from build123d import *

# Parameters (mm, degrees)
SKETCH1_R           = 2.5
BOSS_EXTRUDE1_DEPTH = 3
SKETCH2_W           = 5
SKETCH2_H           = 1
BOSS_EXTRUDE2_DEPTH = 3
CUT_EXTRUDE1_REACH  = 15.032
SKETCH3_W           = 1
SKETCH3_H           = 3.5


with BuildPart() as part:
    # Sketch1 → Boss-Extrude1 (new body)
    with BuildSketch(Plane.XY):
        with BuildLine():
            Line((-6.654411765, -2.5), (-11.654411765, -2.5))
            Line((-11.654411765, -2.5), (-11.654411765, -5))
            Line((-11.654411765, -5), (-5.608785246, -5))
            add(Edge.make_bspline(
                [(-5.608785246, -5), (3.217675956, -4.682890968), (11.654411765, -2.5)],
                knots=[0.187203543, 0.187203543, 0.187203543, 0.737930507, 0.737930507, 0.737930507], degree=2))
            Line((11.654411765, -2.5), (11.654411765, 2.5))
            add(Edge.make_bspline(
                [(-5.608785246, 5), (3.217675956, 4.682890968), (11.654411765, 2.5)],
                knots=[0.187203543, 0.187203543, 0.187203543, 0.737930507, 0.737930507, 0.737930507], degree=2))
            Line((-5.608785246, 5), (-11.654411765, 5))
            Line((-11.654411765, 5), (-11.654411765, 2.5))
            Line((-11.654411765, 2.5), (-6.654411765, 2.5))
            Line((-6.654411765, 2.5), (-6.654411765, -2.5))
        make_face()
        with Locations((6.654411765, 0)):
            Circle(SKETCH1_R, mode=Mode.SUBTRACT)
    extrude(amount=BOSS_EXTRUDE1_DEPTH)

    # Sketch2 → Boss-Extrude2 (add)
    with BuildSketch(Plane.XY.offset(3)):
        with Locations((-9.154411765, 2)):
            Rectangle(SKETCH2_W, SKETCH2_H)
        with Locations((-9.154411765, -2)):
            Rectangle(SKETCH2_W, SKETCH2_H)
    extrude(amount=-BOSS_EXTRUDE2_DEPTH)

    # Sketch3 → Cut-Extrude1 (cut, up to next)
    with BuildSketch(Plane.XY.offset(3), mode=Mode.PRIVATE) as cut_extrude1_sk1:
        with Locations((-11.154411765, 3.25)):
            Rectangle(SKETCH3_W, SKETCH3_H)
    cut_extrude1_tool1 = extrude(cut_extrude1_sk1.sketch, amount=-CUT_EXTRUDE1_REACH, mode=Mode.PRIVATE) & part.part
    # Sketch3 → Cut-Extrude1 (cut, up to next)
    with BuildSketch(Plane.XY.offset(3), mode=Mode.PRIVATE) as cut_extrude1_sk2:
        with Locations((-11.154411765, -3.25)):
            Rectangle(SKETCH3_W, SKETCH3_H)
    cut_extrude1_tool2 = extrude(cut_extrude1_sk2.sketch, amount=-CUT_EXTRUDE1_REACH, mode=Mode.PRIVATE) & part.part
    add(cut_extrude1_tool1.solids().sort_by_distance((-11.154412, 3.25, 3))[0], mode=Mode.SUBTRACT)
    add(cut_extrude1_tool2.solids().sort_by_distance((-11.154412, -3.25, 3))[0], mode=Mode.SUBTRACT)


solid = part.part
Input: part model. Units: mm. Frame: model coordinates. A direction names the side the tool comes from. Round coordinates to 2 decimals unless told otherwise and drop trailing zeros. Order: outer loops, then holes, each group sorted by start corner. A loop starts at its lowest first (then second) coordinate and runs counter-clockwise, first axis right, second up. Notation, with made-up numbers: (78.25, 40.5) - (118.25, 40.5) arc R14 ccw to (118.25, 64.5) - close; hole circle Ø7 at (24, 14). An arc over 180 degrees is marked (long way). Use a Markdown table: item, result.
1. Material intervals for probe 1 along Y at (x, z) = (-7, 2.45); probe 2 along Y at (x, z) = (-5.5, 2.25); probe 3 along X at (y, z) = (2.25, 0.75), sorted ascending.
Evaluation:
| item | result |
|---|---|
| probe 1 | -5 to -1.5, 1.5 to 5 |
| probe 2 | -5 to 5 |
| probe 3 | -10.65 to 5.56, 7.74 to 11.65 |
2. Section B-B on y = 1.25. Return the cut outline in (x, z).
Evaluation:
| item | result |
|---|---|
| outline | (-6.65, 0) - (4.49, 0) - (4.49, 3) - (-6.65, 3) - close; (8.82, 0) - (11.65, 0) - (11.65, 3) - (8.82, 3) - close |
3. Mould query, pull axis Y, two halves, no side actions, for faces 1 (the face through (11.654, 0, 1)), 2 (the face through (-8, -5, 1)), 3 (the face through (-6.654, 0, 1)). Classes: +Y half, -Y half, draft (parallel to the pull), parting line (faces both ways), or undercut.
Evaluation:
| item | result |
|---|---|
| face 1 | draft |
| face 2 | -Y half |
| face 3 | undercut |
4. Access query for faces 4 (the face through (4.157, 0.11, 1.479)), 5 (the face through (-9, -1.5, 2)). Directions: +Z, -Z, +X, -X, +Y, -Y. A direction counts if a zero-diameter tool reaches every point of the face in a straight line with its end or side. Return the directions, or none.
Evaluation:
| item | result |
|---|---|
| face 4 | +Z, -Z |
| face 5 | +Z, -Z, -X |
5. Section A-A on y = 0. Return the cut outline in (x, z), then the cut area to 3 significant figures.
Evaluation:
| item | result |
|---|---|
| outline | (-6.65, 0) - (4.15, 0) - (4.15, 3) - (-6.65, 3) - close; (9.15, 0) - (11.65, 0) - (11.65, 3) - (9.15, 3) - close |
| area | 39.9 mm^2 |
6. First-contact query: pin 1 (1 mm diameter, centred on x = 3.5, z = 1, fed in from +Y). Flat tip, straight axial feed; report the tip coordinate or a pass-through.
Evaluation:
| item | result |
|---|---|
| pin 1 | y = 4.23 |
